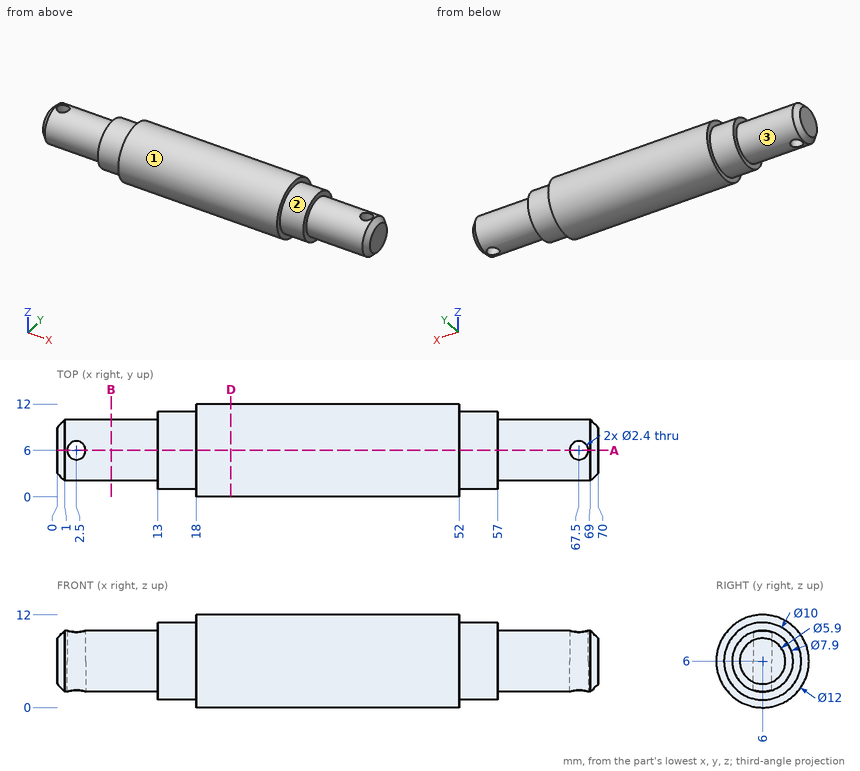
Design review of the part shown in the three views and the two pictorial views. Dimensions are in mm from the part's minimum x, y and z. A direction names the side the tool comes from. Round coordinates to 2 decimals unless told otherwise and drop trailing zeros. Loops run counter-clockwise (first coordinate to the right, second up) from the corner with the lowest first, then second, coordinate; pieces in that order, holes last. Notation, with made-up numbers: (-13.5, 32.5) -> (43.5, 32.5) arc R19 ccw to (43.5, 37.5) -> close; hole circle Ø1 at (34, 57). An arc over 180 degrees is marked (long way). Answer as a JSON object with one key per item and string values. Group by question number.
1) For the marked faces 1, 2 and 3, list the 3-axis set-ups (+Z, -Z, +X, -X, +Y, -Y) from which the entire face can be reached by the end or side of a thin tool; tool diameter is ignored.
2) For line 1 (X direction, y = 6, z = 3.15); line 2 (X direction, y = 5, z = 8.5); line 3 (X direction, y = 3, z = 9.25), list the stretches that pass through material, from the lowest coordinate up. Write a range as [from, to].
3) We need section A-A on y = 6. Give the number of separate pieces and of enclosed holes in the cut face, then the cut area to 3 significant figures.
4) We need section D-D on x = 22.5. Write out the cut boundary in (y, z), then the cut area to 3 significant figures.
5) For pin 1 Ø6 at (x, z) = (41, 10) entering from -Y; pin 2 Ø3 at (x, y) = (2.5, 6) entering from +Z; pin 3 Ø1 at (x, z) = (15.5, 7.5) entering from -Y, all flat-tipped, find the tip position at first contact; note any pin that passes through.
6) We need section B-B on x = 7. Write out the cut boundary in (y, z).
Result set:
{
 "1": {"face 1": "+X, -X", "face 2": "+X", "face 3": "-X"},
 "2": {"line 1": "[0, 1.3], [3.7, 66.3], [68.7, 70]", "line 2": "[0, 1.84], [3.16, 66.84], [68.16, 70]", "line 3": "[13, 57]"},
 "3": {"separate pieces": "3", "enclosed holes": "0", "area": "673 mm²"},
 "4": {"outline": "circle Ø12 at (6, 6)", "area": "113 mm²"},
 "5": {"pin 1": "y = 0.08", "pin 2": "z = 9.95", "pin 3": "y = 1.1"},
 "6": {"outline": "circle Ø7.9 at (6, 6)"}
}
